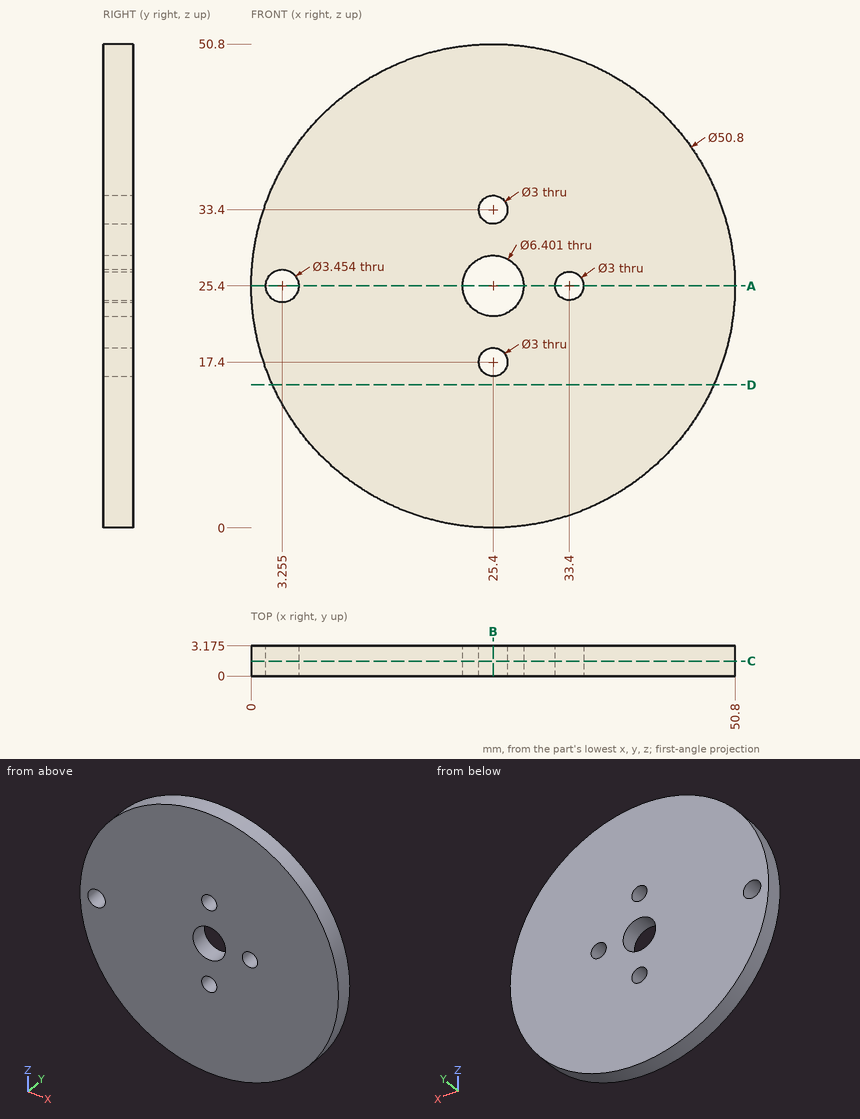
Geometry check sheet. Reference: drawing and pictorial views, mm from the part's lowest x, y, z. Round coordinates to 2 decimals unless told otherwise and drop trailing zeros. Order: outer loops, then holes, each group sorted by start corner. A loop starts at its lowest first (then second) coordinate and runs counter-clockwise, first axis right, second up. Notation, with made-up numbers: M -31,-21 L -17,-21 A23 cw -17,3 Z; hole C -17,40 d4. An arc over 180 degrees is marked long. Answer in a Markdown table with one row per item.
(1) Sectioned sample at D-D, the plane z = 15. Record the cut outline in (x, y) (1 decimal), and give its area (3 significant figures).
Responses:
| item | result |
|---|---|
| outline | M 2.2,0 L 48.6,0 L 48.6,3.2 L 2.2,3.2 Z |
| area | 147 mm² |
(2) Sectioned sample at B-B, the plane x = 25.4. Record the cut outline in (y, z) (1 decimal).
Responses:
| item | result |
|---|---|
| outline | M 0,0 L 3.2,0 L 3.2,15.9 L 0,15.9 Z; M 0,18.9 L 3.2,18.9 L 3.2,22.2 L 0,22.2 Z; M 0,28.6 L 3.2,28.6 L 3.2,31.9 L 0,31.9 Z; M 0,34.9 L 3.2,34.9 L 3.2,50.8 L 0,50.8 Z |
(3) Sectioned sample at C-C, the plane y = 1.55. Record the cut outline in (x, z) (1 decimal), and give its area (3 significant figures).
Responses:
| item | result |
|---|---|
| outline | C 25.4,25.4 d50.8; hole C 3.3,25.4 d3.5; hole C 25.4,25.4 d6.4; hole C 25.4,17.4 d3; hole C 25.4,33.4 d3; hole C 33.4,25.4 d3 |
| area | 1,960 mm² |
(4) Sectioned sample at A-A, the plane z = 25.4. Record the cut outline in (x, y) (1 decimal).
Responses:
| item | result |
|---|---|
| outline | M 0,0 L 1.5,0 L 1.5,3.2 L 0,3.2 Z; M 5,0 L 22.2,0 L 22.2,3.2 L 5,3.2 Z; M 28.6,0 L 31.9,0 L 31.9,3.2 L 28.6,3.2 Z; M 34.9,0 L 50.8,0 L 50.8,3.2 L 34.9,3.2 Z |
(5) Go/stop test with flat-tipped pins: P1, Ø1, axis at y = 2, z = 16.5, coming from the -X side; P2, Ø3, axis at x = 3.26, z = 25.4, coming from the -Y side. Record where each tip stops, or that it passes through.
Responses:
| item | result |
|---|---|
| P1 | stops at x = 1.43 |
| P2 | passes through |
(6) Scan lines: probe 1 along Z at (x, y) = (25.4, 2.3); probe 2 along X at (y, z) = (0.8, 25.4); probe 3 along X at (y, z) = (1.95, 33) (1 decimal). Record each from-to range of solid material in increasing order. Write a range as from..to.
Responses:
| item | result |
|---|---|
| probe 1 | z = 0..15.9, 18.9..22.2, 28.6..31.9, 34.9..50.8 |
| probe 2 | x = 0..1.53, 4.98..22.2, 28.6..31.9, 34.9..50.8 |
| probe 3 | x = 1.2..24, 26.8..49.6 |
